Autodesk Inventor part; units mm, degrees
ref_plane "YZ Plane" through (0, 0, 0) normal (1, 0, 0) x (0, 1, 0)
ref_plane "XZ Plane" through (0, 0, 0) normal (0, 1, 0) x (-1, 0, 0)
ref_plane "XY Plane" through (0, 0, 0) normal (0, 0, 1) x (1, 0, 0)
sketch "Sketch1" plane through (0, 0, 0) normal (0, 0, 1) x (1, 0, 0)
  circle A0 centre (0, 0) radius 16.51
  circle A1 centre (0, 0) radius 8.255
  dimension "d0" = 33.02
  dimension "d3" = 16.51
extrude "Extrusion2" add sketch "Sketch1" along normal blind 11.43
sketch "Sketch2" plane through (0, 0, 11.43) normal (0, 0, 1) x (1, 0, 0)
  circle A0 centre (0, 0) radius 12.065
  circle A1 centre (0, 0) radius 12.319
  circle A2 centre (0, 0) radius 8.255
  dimension "d6" = 0.254
  dimension "d8" = 3.81
extrude "Extrusion3" cut sketch "Sketch2" against normal blind 0.254 contours A1
properties part number "RobotArm ShaftColar"
The listing builds one solid part. Answer for the finished solid, in the listing's coordinates (mm). Coordinates: 2 decimals unless noted, no trailing zeros. Write each loop counter-clockwise with the first axis right and the second up, starting at its lowest first coordinate (ties: lowest second). Pieces come first, ordered by that corner, then holes. Notation, with made-up numbers: (0.5, -39.5) - (52.5, -39.5) arc R35 ccw to (52.5, -7.5) - close; hole circle Ø6 at (43, 75). An arc over 180 degrees is marked (long way). Answer as CSV lines item,"result".
1. Find section A-A (x = 0). Give the vertices of the cut face in (y, z) (3 decimals), plus the area to 3 significant figures.
Computed values:
outline,"(-16.51, 0) - (-8.255, 0) - (-8.255, 11.43) - (-12.065, 11.43) - (-12.065, 11.176) - (-12.319, 11.176) - (-12.319, 11.43) - (-16.51, 11.43) - close; (8.255, 0) - (16.51, 0) - (16.51, 11.43) - (12.319, 11.43) - (12.319, 11.176) - (12.065, 11.176) - (12.065, 11.43) - (8.255, 11.43) - close"
area,"189 mm²"
2. Find section D-D (y = -10.5). Give the vertices of the cut face in (x, z).
Computed values:
outline,"(-12.74, 0) - (12.74, 0) - (12.74, 11.43) - (6.44, 11.43) - (6.44, 11.18) - (5.94, 11.18) - (5.94, 11.43) - (-5.94, 11.43) - (-5.94, 11.18) - (-6.44, 11.18) - (-6.44, 11.43) - (-12.74, 11.43) - close"
3. Given P1, Ø4, axis at y = 12, z = 5, coming from the +X side; P2, Ø4, axis at x = -11.5, z = 6.5, coming from the -Y side; P3, Ø1, axis at x = -4.5, z = 4, coming from the +Y side, each flat-ended and moving along its own axis, determine where each tip first touches the part or whether it passes through.
Computed values:
P1,"stops at x = 13.14"
P2,"stops at y = -13.5"
P3,"stops at y = 16.02"
4. Straight lines are drawn through the part: line 1 (Y direction, x = 0, z = 11.3) (3 decimals); line 2 (Y direction, x = 0, z = 3.75) (3 decimals); line 3 (Y direction, x = -10.5, z = 11.25). For each, find the intervals that lie inside material, in ascending order. Write a range as [from, to].
Computed values:
line 1,"y = [-16.51, -12.319], [-12.065, -8.255], [8.255, 12.065], [12.319, 16.51]"
line 2,"y = [-16.51, -8.255], [8.255, 16.51]"
line 3,"y = [-12.74, -6.44], [-5.94, 5.94], [6.44, 12.74]"
5. Determine the mould class of faces 1 (the flat face through (3, -8, 11.43)), 2 (the cylindrical face through (15.748, -4.959, 5.635)), 3 (the cylindrical face through (7.874, -2.48, 5.635)) for opening direction X: +X half, -X half, draft (parallel to the pull), parting line (faces both ways), or undercut.
Computed values:
face 1,"draft"
face 2,"parting line"
face 3,"undercut"
6. Find section C-C (z = 8). Give the vertices of the cut face in (x, y) (3 decimals).
Computed values:
outline,"circle Ø33.02 at (0, 0); hole circle Ø16.51 at (0, 0)"
